Read the model definition and answer for the solid it produces. Units are mm, in the model's axes. A direction names the side the tool comes from. Round coordinates to 2 decimals unless told otherwise and drop trailing zeros. Loops run counter-clockwise (first coordinate to the right, second up) from the corner with the lowest first, then second, coordinate; pieces in that order, holes last. Notation, with made-up numbers: M 11.5,72 L 67.5,72 A26 ccw 67.5,102 Z; hole C 39.25,-36.75 d11. An arc over 180 degrees is marked long. Write each question's results on one line, items separated by ' | '.
Autodesk Inventor part; units mm, degrees
ref_plane "YZ Plane" through (0, 0, 0) normal (1, 0, 0) x (0, 1, 0)
ref_plane "XZ Plane" through (0, 0, 0) normal (0, 1, 0) x (-1, 0, 0)
ref_plane "XY Plane" through (0, 0, 0) normal (0, 0, 1) x (1, 0, 0)
sketch "Sketch1" plane through (0, 0, 0) normal (0, 1, 0) x (-1, 0, 0)
  line L0 (0, 0) -> (-200, 0)
  line L1 (-200, 0) -> (-200, -200)
  line L2 (-200, -200) -> (0, -200)
  line L3 (0, -200) -> (0, 0)
  line L4 (-89.8726, -200) -> (-110.1274, -200)
  line L5 (-114.7696, -186.0054) -> (-100, -186.0054)
  line L6 (-110.1274, -200) -> (-115.8572, -187.7125)
  arc A0 (-114.7696, -186.0054) -> (-115.8572, -187.7125) centre (-114.7696, -187.2054) ccw
  line L7 (-100, -186.0054) -> (-85.2304, -186.0054)
  line L8 (-90, -199.8) -> (-90, -186.3697) construction
  arc A1 (-84.1428, -187.7125) -> (-85.2304, -186.0054) centre (-85.2304, -187.2054) ccw
  line L9 (-84.1428, -187.7125) -> (-89.8726, -200)
  line L10 (-0.2, -90) -> (13.2303, -90) construction
  arc A2 (12.0565, -115.4946) -> (13.1946, -114.7696) centre (12.3946, -114.7696) ccw
  line L11 (0, -109.8726) -> (12.0565, -115.4946)
  line L12 (0, -90.1274) -> (0, -109.8726)
  line L13 (13.1946, -114.7696) -> (13.1946, -100)
  line L14 (12.0565, -84.5054) -> (0, -90.1274)
  line L15 (13.1946, -100) -> (13.1946, -85.2304)
  arc A3 (13.1946, -85.2304) -> (12.0565, -84.5054) centre (12.3946, -85.2304) ccw
  point P0 (-100, -200)
  point P1 (-100, -200)
  point P2 (-100, -200)
  point P3 (-83.6607, -186.2054)
  point P4 (-100, -200)
  point P5 (0, -100)
  point P6 (0, -100)
  point P7 (0, -100)
  point P8 (0, -100)
  point P9 (0, -100)
  point P10 (0, -100)
  dimension "d0" = 200
  dimension "d1" = 200
  dimension "d2" = 15
extrude "Extrusion1" add sketch "Sketch1" along normal blind 60 contours L3 L2 L9 A1 L7 L5 A0 L6 L1 L0 | L6 A0 L5 L7 A1 L9 L2
extrude "Extrusion3" cut sketch "Sketch1" along normal blind 5.2 contours L6 A0 L5 L7 A1 L9 L2
sketch "Sketch2" plane through (0, 60, 0) normal (0, 1, 0) x (1, 0, 0)
  point P0 (0, 0)
sketch "Sketch3" plane through (0, 60, 0) normal (0, 1, 0) x (1, 0, 0)
  line L0 (0, 0) -> (200, 0)
  circle A0 centre (100, 75) radius 5.1
  line L1 (200, 200) -> (0, 200)
  circle A1 centre (100, 200) radius 5.1
  dimension "d10" = 10.2
  dimension "d11" = 10.2
extrude "Extrusion4" cut sketch "Sketch3" against normal blind 5.2
extrude "Extrusion5" add sketch "Sketch1" along normal blind 4.8 contours L14 A3 L15 L13 A2 L11 L3
sketch "Sketch4" plane through (0, 60, 0) normal (0, 1, 0) x (1, 0, 0)
  line L0 (0, 200) -> (0, 0)
  line L1 (200, 0) -> (200, 200)
  line L2 (0, 0) -> (200, 0)
  line L3 (200, 0) -> (200, 50)
  line L4 (200, 50) -> (0, 50)
  line L5 (0, 50) -> (0, 0)
  line L6 (200, 200) -> (110.1274, 200)
  line L7 (200, 0) -> (130, 0)
  line L8 (130, 0) -> (130, 200)
  line L9 (130, 200) -> (200, 200)
  line L10 (200, 200) -> (200, 0)
  point P0 (130, 50)
  dimension "d16" = 50
  dimension "d17" = 70
extrude "Extrusion6" cut sketch "Sketch4" against normal blind 60
sketch "Sketch5" plane through (0, 0, 0) normal (0, -1, 0) x (1, 0, 0)
  line L0 (89.8726, -200) -> (0, -200)
  line L1 (0, -200) -> (70, -200)
  line L2 (70, -200) -> (70, -120)
  line L3 (70, -120) -> (0, -120)
  line L4 (0, -120) -> (0, -200)
  point P0 (0, 0)
  dimension "d20" = 70
  dimension "d21" = 80
extrude "Extrusion7" cut sketch "Sketch5" against normal blind 60
sketch "Sketch6" plane through (130, 60, -50) normal (1, 0, 0) x (0, 0, -1)
  line L0 (0, 0) -> (0, -60)
  line L1 (150, -60) -> (0, -60)
  line L2 (0, 0) -> (150, 0)
  line L3 (150, 0) -> (150, -60)
  line L4 (150, -60) -> (0, -60)
  line L5 (0, -60) -> (0, 0)
  point P0 (-50, -60)
extrude "Extrusion8" add sketch "Sketch6" along normal blind 20
fillet "Fillet2" radius 10 6 edges at (150, 30, -200) (70, 30, -200) (0, 30, -120) (150, 30, -50) (70, 30, -120) (0, 30, -50)
properties part number "Area øh1"
Item 1: Straight lines are drawn through the part: line 1 (Z direction, x = 100, y = 56); line 2 (X direction, y = 58.05, z = -75); line 3 (X direction, y = 17, z = -161). For each, find the intervals that lie inside material, in ascending order.
Outcome:
line 1: z = -194.9 to -80.1, -69.9 to -50 | line 2: x = 0 to 94.9, 105.1 to 150 | line 3: x = 70 to 150
Item 2: The mould has two halves that part along Z. Classify faces 1 (the face through (-5.944, 2.366, -112.644)), 2 (the face through (0, 30, -85)), 3 (the face through (86.968, 2.564, -193.77)): pulls with the +Z half, pulls with the -Z half, needs draft (parallel to the pull), parting line crosses it, or undercut.
Outcome:
face 1: pulls with the -Z half | face 2: needs draft | face 3: undercut
Item 3: For faces 4 (the face through (96.2, 57.4, -78.4)), 5 (the face through (-6.11, 2.37, -87.28)), 6 (the face through (100, 3, -186.005)), 7 (the face through (100, 54.8, -198)), 8 (the face through (35, 30, -120)), determine the directions among +Z, -Z, +X, -X, +Y, -Y from which every point of the face is accessible in a straight line to the end or side of a thin tool.
Outcome:
face 4: +Y | face 5: +Z, +Y, -Y | face 6: -Y | face 7: -Z, +Y | face 8: -Z, -X, +Y, -Y
Item 4: The part is cut by section A-A (x = 100). Determine the outline of the cut face in (y, z), plus the area to 3 significant figures.
Outcome:
outline: M 0,-186.01 L 5.2,-186.01 L 5.2,-200 L 54.8,-200 L 54.8,-194.9 L 60,-194.9 L 60,-80.1 L 54.8,-80.1 L 54.8,-69.9 L 60,-69.9 L 60,-50 L 0,-50 Z | area: 8,850 mm2
Item 5: The part is cut by section B-B (y = 27.5). Determine the outline of the cut face in (x, z).
Outcome:
outline: M 0,-110 A10 ccw 10,-120 L 60,-120 A10 cw 70,-130 L 70,-190 A10 ccw 80,-200 L 140,-200 A10 ccw 150,-190 L 150,-60 A10 ccw 140,-50 L 10,-50 A10 ccw 0,-60 Z
Item 6: The part is cut by section C-C (z = -75). Determine the outline of the cut face in (x, y).
Outcome:
outline: M 0,0 L 150,0 L 150,60 L 105.1,60 L 105.1,54.8 L 94.9,54.8 L 94.9,60 L 0,60 Z
Item 7: Flat-ended cylindrical pins translate along their axes: pin 1 (4 mm diameter, centred on x = 98, y = 1.5, fed in from -Z); pin 2 (8 mm diameter, centred on x = 100, z = -75, fed in from +Y); pin 3 (6.5 mm diameter, centred on x = -7, z = -94.5, fed in from +Y). Find the tip coordinate at first contact, or state that the pin passes through.
Outcome:
pin 1: stops at z = -186.01 | pin 2: stops at y = 54.8 | pin 3: stops at y = 4.8
Item 8: The part is cut by section D-D (x = 30.5). Determine the outline of the cut face in (y, z), plus the area to 3 significant figures.
Outcome:
outline: M 0,-120 L 60,-120 L 60,-50 L 0,-50 Z | area: 4,200 mm2
